The listing builds one solid part. Answer for the finished solid, in the listing's coordinates (mm). A direction names the side the tool comes from. Coordinates: 2 decimals unless noted, no trailing zeros. Loops run counter-clockwise (first coordinate to the right, second up) from the corner with the lowest first, then second, coordinate; pieces in that order, holes last. Notation, with made-up numbers: M 87.5,29.5 L 92.5,29.5 A30 cw 92.5,56.5 Z; hole C -27,81.25 d2. An arc over 180 degrees is marked long. Return JSON: item names as keys, results as strings. Group by question number.
1. Straight lines are drawn through the part: L1, parallel to Y at x = 13.5, z = 9.5; L2, parallel to Z at x = 15, y = 7.5; L3, parallel to Z at x = -13, y = 7. For each, find the intervals that lie inside material, in ascending order. Write a range as from..to.
2. Section A-A (z = -6) is taken. Write down the section's boundary in (x, y).
3. Which of the six approach directions +Z, -Z, +X, -X, +Y, -Y give full straight-line access (tool end or side, diameter ignored) to faces 4 (the face through (16.63, 13.73, -17.27)), 5 (the face through (11.5, -1, -13)), 6 (the face through (0, -1, 19.5))?
4. The mould has two halves that part along X. Classify faces 1 (the face through (-16, 15, -16)), 2 (the face through (19.5, -1, 0)), 3 (the face through (-14.37, 13.73, -17.27)): pulls with the +X half, pulls with the -X half, needs draft (parallel to the pull), parting line crosses it, or undercut.
5. Section D-D (z = 9) is taken. Write down the section's boundary in (x, y).
6. Given P1, Ø10.5, axis at x = 9.5, z = 4.5, coming from the +Y side, flat-ended and moving along its own axis, determine where the tip first touches the part or whether it passes through.
7. Section B-B (y = 1) is taken. Write down the section's boundary in (x, z).
8. Section C-C (x = 0) is taken. Write down the section's boundary in (y, z).
```python
from build123d import *

# Parameters (mm, degrees)
SKETCH1_R             = 4
BOSS_EXTRUDE1_DEPTH   = 12.5
BOSS_EXTRUDE1_2_DEPTH = 12.5
BOSS_EXTRUDE1_3_DEPTH = 12.5
BOSS_EXTRUDE1_4_DEPTH = 12.5
SKETCH2_R             = 2.1
BOSS_EXTRUDE2_DEPTH   = 2.5
BOSS_EXTRUDE3_DEPTH   = 2


with BuildPart() as part:
    # Sketch1 → Boss-Extrude1 (new body)
    with BuildSketch(Plane(origin=(0, 0, 0), x_dir=(1, 0, 0), z_dir=(0, 1, 0))):
        with Locations((-15.5, -15.5)):
            Circle(SKETCH1_R)
    extrude(amount=BOSS_EXTRUDE1_DEPTH)



with BuildPart() as body_2:
    # Sketch1 → Boss-Extrude1 2 (new body)
    with BuildSketch(Plane(origin=(0, 0, 0), x_dir=(1, 0, 0), z_dir=(0, 1, 0))):
        with Locations((-15.5, 15.5)):
            Circle(SKETCH1_R)
    extrude(amount=BOSS_EXTRUDE1_2_DEPTH)


with BuildPart() as body_3:
    # Sketch1 → Boss-Extrude1 3 (new body)
    with BuildSketch(Plane(origin=(0, 0, 0), x_dir=(1, 0, 0), z_dir=(0, 1, 0))):
        with Locations((15.5, -15.5)):
            Circle(SKETCH1_R)
    extrude(amount=BOSS_EXTRUDE1_3_DEPTH)


with BuildPart() as body_4:
    # Sketch1 → Boss-Extrude1 4 (new body)
    with BuildSketch(Plane(origin=(0, 0, 0), x_dir=(1, 0, 0), z_dir=(0, 1, 0))):
        with Locations((15.5, 15.5)):
            Circle(SKETCH1_R)
    extrude(amount=BOSS_EXTRUDE1_4_DEPTH)


with BuildPart() as part_1:
    add(part.part)

    add(body_2.part)  # Boss-Extrude2 merges body 2

    add(body_3.part)  # Boss-Extrude2 merges body 3

    add(body_4.part)  # Boss-Extrude2 merges body 4
    # Sketch2 → Boss-Extrude2 (add)
    with BuildSketch(Plane(origin=(0, 12.5, 0), x_dir=(1, 0, 0), z_dir=(0, 1, 0))):
        with Locations((-15.5, 15.5)):
            Circle(SKETCH2_R)
        with Locations((15.5, 15.5)):
            Circle(SKETCH2_R)
        with Locations((15.5, -15.5)):
            Circle(SKETCH2_R)
        with Locations((-15.5, -15.5)):
            Circle(SKETCH2_R)
    extrude(amount=BOSS_EXTRUDE2_DEPTH)

    # Sketch3 → Boss-Extrude3 (add)
    with BuildSketch(Plane.XZ):
        with BuildLine():
            Line((-19.5, 15.5), (-19.5, -15.5))
            ThreePointArc((-19.5, -15.5), (-18.328427125, -18.328427125), (-15.5, -19.5))
            ThreePointArc((-15.5, -19.5), (-12.671572875, -18.328427125), (-11.5, -15.5))
            Line((-11.5, -15.5), (-11.5, -10.496545835))
            ThreePointArc((-11.5, -10.496545835), (0, 1.003454165), (11.5, -10.496545835))
            Line((11.5, -10.496545835), (11.5, -15.5))
            ThreePointArc((11.5, -15.5), (12.671572875, -18.328427125), (15.5, -19.5))
            ThreePointArc((15.5, -19.5), (18.328427125, -18.328427125), (19.5, -15.5))
            Line((19.5, -15.5), (19.5, 15.5))
            ThreePointArc((19.5, 15.5), (18.328427125, 18.328427125), (15.5, 19.5))
            Line((15.5, 19.5), (-15.5, 19.5))
            ThreePointArc((-15.5, 19.5), (-18.328427125, 18.328427125), (-19.5, 15.5))
        make_face()
    extrude(amount=BOSS_EXTRUDE3_DEPTH)


solid = part_1.part
```
Worked out:
{
 "1": {"L1": "-2..0", "L2": "-19.47..-11.53, 11.53..19.47", "L3": "-18.62..-12.38, 12.38..18.62"},
 "2": {"outline": "M -19.5,-2 L -10.58,-2 L -10.58,0 L -19.5,0 Z; M 10.58,-2 L 19.5,-2 L 19.5,0 L 10.58,0 Z"},
 "3": {"face 4": "+Y", "face 5": "-Z, +Y, -Y", "face 6": "+Z, +X, -X, +Y, -Y"},
 "4": {"face 1": "needs draft", "face 2": "pulls with the +X half", "face 3": "undercut"},
 "5": {"outline": "M -19.5,-2 L 19.5,-2 L 19.5,0 L -19.5,0 Z"},
 "6": {"P1": "y = 0"},
 "7": {"outline": "C -15.5,-15.5 d8; C -15.5,15.5 d8; C 15.5,-15.5 d8; C 15.5,15.5 d8"},
 "8": {"outline": "M -2,1 L 0,1 L 0,19.5 L -2,19.5 Z"}
}
